from build123d import *

# Parameters (mm, degrees)
F0_W     = 143.9583450556
F0_H     = 95.0037688017
F1_DEPTH = 12.446
F2_R     = 55.2801974118
F3_DEPTH = 61.722
F4_R     = 36.192071595
F5_DEPTH = 61.723
F7_DEPTH = 7.112


with BuildPart() as f1:
    # F0 (on Top) → F1 (new body)
    with BuildSketch(Plane.XY):
        Rectangle(F0_W, F0_H)
    extrude(amount=F1_DEPTH)

    # F2 (on Top) → F3 (join)
    with BuildSketch(Plane.XY):
        with Locations((55.2801974118, 0)):
            Circle(F2_R)
    extrude(amount=F3_DEPTH)

    # F4 (on face) → F5 (cut, through all)
    with BuildSketch(Plane.XY.offset(61.722)):
        with Locations((55.2801974118, 0)):
            Circle(F4_R)
    extrude(amount=-F5_DEPTH, mode=Mode.SUBTRACT)

    # F6 (on Front) → F7 (join, symmetric)
    with BuildSketch(Plane.XZ):
        Polygon((9.263087064, 7.2733671404), (9.263087064, 56.0136325657), (-61.6970062256, 7.2733671404), align=None)
    extrude(amount=F7_DEPTH, both=True)


solid = f1.part
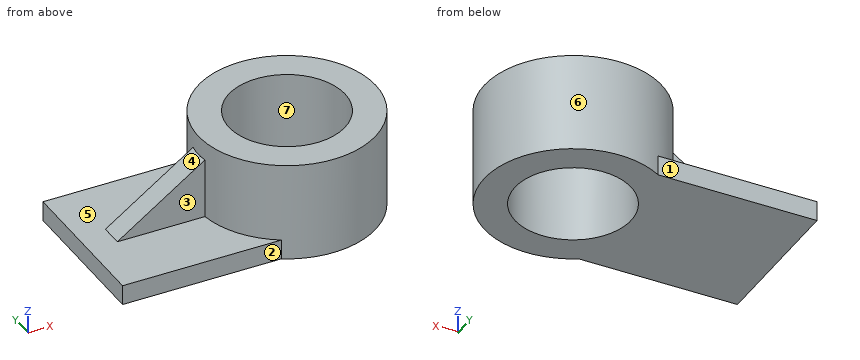
Can you work these out from the model? Positions are in its coordinate system, mm. Face numbers are marked on the shaded views. A direction names the side the tool comes from. Round coordinates to 2 decimals unless told otherwise and drop trailing zeros. Write each loop counter-clockwise with the first axis right and the second up, starting at its lowest first coordinate (ties: lowest second). Pieces come first, ordered by that corner, then holes. Notation, with made-up numbers: M 60.5,-20.5 L 75.5,-20.5 A17 cw 75.5,-4.5 Z; hole C 74.25,32 d10. An arc over 180 degrees is marked long. Use CSV: the item, a comma, the result in double quotes.
(1) On a 3-axis mill with a long thin cutter (end or side, diameter ignored), from which of +Z, -Z, +X, -X, +Y, -Y can I reach the whole of each face in a straight line? I mean the marked faces 1, 2 and 3. Say none if no direction works.
Check values:
face 1,"+Z, -Z, -X, +Y"
face 2,"+Z, -Z, -X, -Y"
face 3,"+Z, -X, -Y"
(2) Imagine slicing it at B-B (z = 9.5). Write out the boundary of the cut face in (x, y), plus the area to 3 significant figures.
Check values:
outline,"M -71.98,-47.5 L 27.01,-47.5 A55.28 ccw long 27.01,47.5 L -71.98,47.5 Z; hole C 55.28,0 d72.38"
area,"13,100 mm^2"
(3) We'd pull the mould along X, two halves only. Please class the marked faces 4, 5, 6 and 7: +X half, -X half, draft (parallel to the pull), parting line (faces both ways), or undercut.
Check values:
face 4,"-X half"
face 5,"draft"
face 6,"parting line"
face 7,"undercut"
(4) Imagine slicing it at C-C (x = 37). Write out the boundary of the cut face in (y, z).
Check values:
outline,"M -52.17,0 L -31.24,0 L -31.24,61.72 L -52.17,61.72 Z; M 31.24,0 L 52.17,0 L 52.17,61.72 L 31.24,61.72 Z"
(5) Imagine slicing it at A-A (y = -29). Write out the boundary of the cut face in (x, z).
Check values:
outline,"M -71.98,0 L 33.63,0 L 33.63,61.72 L 8.22,61.72 L 8.22,12.45 L -71.98,12.45 Z; M 76.93,0 L 102.34,0 L 102.34,61.72 L 76.93,61.72 Z"
(6) I need wall thicknesses on line 1 along Y through (x, z) = (30, 16.5); line 2 along Y through (x, z) = (51, 41.5); line 3 along X through (y, z) = (-20, 23). Which ranges of each line are inside material? Lowest first, please.
Check values:
line 1,"-49.16 to -25.9, 25.9 to 49.16"
line 2,"-55.11 to -35.94, 35.94 to 55.11"
line 3,"3.74 to 25.12, 85.44 to 106.82"
(7) Imagine slicing it at D-D (x = -7.5). Write out the boundary of the cut face in (y, z), plus the area to 3 significant figures.
Check values:
outline,"M -47.5,0 L 47.5,0 L 47.5,12.45 L 7.11,12.45 L 7.11,44.5 L -7.11,44.5 L -7.11,12.45 L -47.5,12.45 Z"
area,"1,640 mm^2"
(8) I'm going to push flat-ended pins straight in: pin 1 (2 mm diameter, centred on y = 22.5, z = 13, fed in from +X); pin 2 (2 mm diameter, centred on x = -17.5, z = 30.5, fed in from +Y); pin 3 (6 mm diameter, centred on x = -46.5, z = 5, fed in from -Y). Where does each tip first touch, or does it pass through?
Check values:
pin 1,"x = 106.21"
pin 2,"y = 7.11"
pin 3,"y = -47.5"
